Drawing for the job (mm, zero at the part's lowest x, y, z). A direction names the side the tool comes from. Coordinates: 2 decimals unless noted, no trailing zeros. Write each loop counter-clockwise with the first axis right and the second up, starting at its lowest first coordinate (ties: lowest second). Pieces come first, ordered by that corner, then holes. Notation, with made-up numbers: M -36.75,75 L -12.75,75 A33 ccw -12.75,110 Z; hole C -37,41 d3. An arc over 180 degrees is marked long. Put each result on its own line as item: value. Start each with the question number.
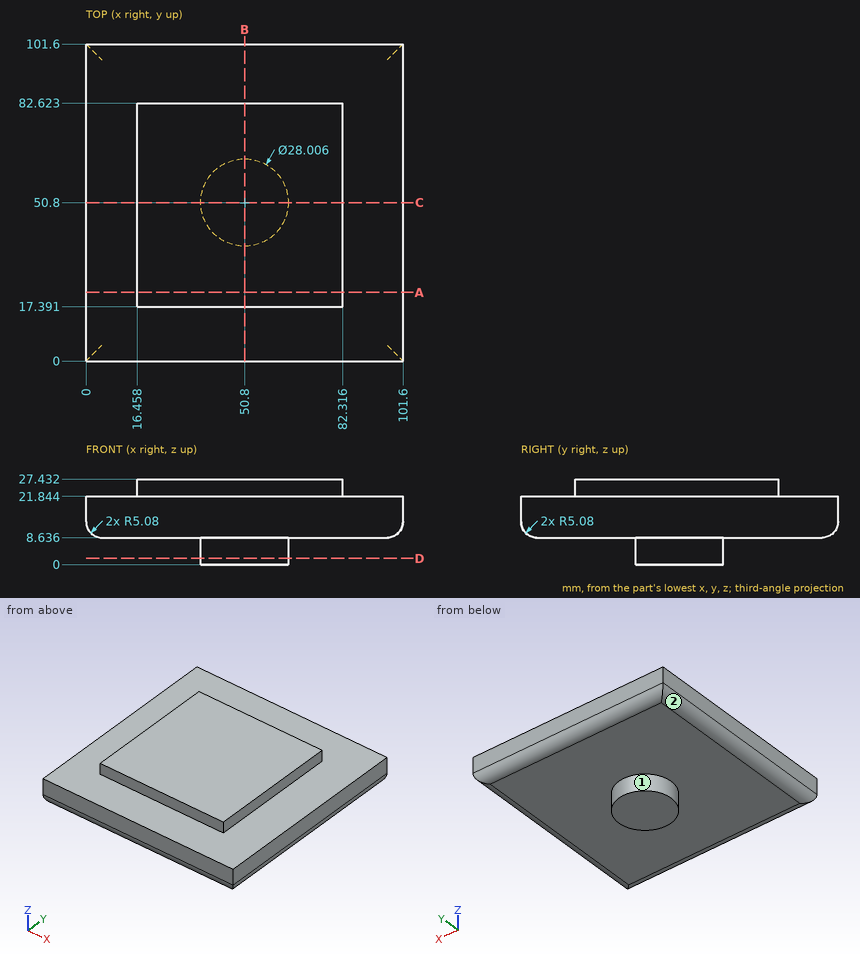
(1) Slice it at A-A, the plane y = 22. Write the cut outline in (x, z).
(2) Drop flat-ended pins along their axis: pin 1 (12 mm diameter, centred on x = 51, y = 81, fed in from -Z); pin 2 (8 mm diameter, centred on x = 12, y = 15.5, fed in from +Z); pin 3 (2 mm diameter, centred on x = 19.5, z = 10, fed in from +Y). Give the stop position or say it passes through.
(3) Slice it at C-C, the plane y = 50.8. Write the cut outline in (x, z).
(4) Slice it at B-B, the plane x = 50.8. Write the cut outline in (y, z).
(5) Slice it at D-D, the plane z = 2. Write the cut outline in (x, y) (1 decimal), then the cut area to 3 significant figures.
(6) Drill centre lines: line 1 (Z direction, x = 90.5, y = 84); line 2 (Z direction, x = 56, y = 71); line 3 (X direction, y = 19.5, z = 24.75). Where is each one in solid material? Low to high. Write a range as [from, to].
(7) Which spindle directions (+Z, -Z, +X, -X, +Y, -Y) get a long thin tool onto all of the face, cutting with end or side? Do the marked faces 1 and 2. Say none if no direction does.
Result set:
1. outline: M 0,13.72 A5.08 ccw 5.08,8.64 L 96.52,8.64 A5.08 ccw 101.6,13.72 L 101.6,21.84 L 82.32,21.84 L 82.32,27.43 L 16.46,27.43 L 16.46,21.84 L 0,21.84 Z
2. pin 1: stops at z = 8.64
2. pin 2: stops at z = 21.84
2. pin 3: stops at y = 100.81
3. outline: M 0,13.72 A5.08 ccw 5.08,8.64 L 36.8,8.64 L 36.8,0 L 64.8,0 L 64.8,8.64 L 96.52,8.64 A5.08 ccw 101.6,13.72 L 101.6,21.84 L 82.32,21.84 L 82.32,27.43 L 16.46,27.43 L 16.46,21.84 L 0,21.84 Z
4. outline: M 0,13.72 A5.08 ccw 5.08,8.64 L 36.8,8.64 L 36.8,0 L 64.8,0 L 64.8,8.64 L 96.52,8.64 A5.08 ccw 101.6,13.72 L 101.6,21.84 L 82.62,21.84 L 82.62,27.43 L 17.39,27.43 L 17.39,21.84 L 0,21.84 Z
5. outline: C 50.8,50.8 d28
5. area: 616 mm^2
6. line 1: z = [8.64, 21.84]
6. line 2: z = [8.64, 27.43]
6. line 3: x = [16.46, 82.32]
7. face 1: -Z
7. face 2: -Z, -X, +Y, -Y
